Build history of the part. All positions in model axes, mm. Face numbers are marked on the shaded views. A direction names the side the tool comes from. Round coordinates to 2 decimals unless told otherwise and drop trailing zeros. Loops run counter-clockwise (first coordinate to the right, second up) from the corner with the lowest first, then second, coordinate; pieces in that order, holes last.
from build123d import *

# Parameters (mm, degrees)
SKETCH1_W           = 6
SKETCH1_H           = 5
BOSS_EXTRUDE1_DEPTH = 8
SKETCH3_W           = 2
SKETCH3_H           = 5
CUT_EXTRUDE1_DEPTH  = 2
SKETCH4_W           = 2
SKETCH4_H           = 2
CUT_EXTRUDE2_DEPTH  = 1
SKETCH5_W           = 6
SKETCH5_H           = 5
CUT_EXTRUDE3_DEPTH  = 2
SKETCH6_W           = 2
SKETCH6_H           = 2
CUT_EXTRUDE4_DEPTH  = 2
CUT_EXTRUDE5_DEPTH  = 1
SKETCH8_W           = 8.535402973
SKETCH8_H           = 3.487061374
CUT_EXTRUDE6_DEPTH  = 1
SKETCH9_W           = 2
SKETCH9_H           = 1
CUT_EXTRUDE7_DEPTH  = 1


with BuildPart() as part:
    # Sketch1 → Boss-Extrude1 (new body)
    with BuildSketch(Plane.XY):
        Rectangle(SKETCH1_W, SKETCH1_H)
    extrude(amount=BOSS_EXTRUDE1_DEPTH)

    # Sketch3 → Cut-Extrude1 (cut)
    with BuildSketch(Plane.XY.offset(8)):
        with Locations((2, 0)):
            Rectangle(SKETCH3_W, SKETCH3_H)
    extrude(amount=-CUT_EXTRUDE1_DEPTH, mode=Mode.SUBTRACT)

    # Sketch4 → Cut-Extrude2 (cut)
    with BuildSketch(Plane.XY.offset(8)):
        with Locations((0, 1.5)):
            Rectangle(SKETCH4_W, SKETCH4_H)
    extrude(amount=-CUT_EXTRUDE2_DEPTH, mode=Mode.SUBTRACT)

    # Sketch5 → Cut-Extrude3 (cut)
    with BuildSketch(Plane(origin=(0, 2.5, 0), x_dir=(1, 0, 0), z_dir=(0, 1, 0))):
        with Locations((0, -3.5)):
            Rectangle(SKETCH5_W, SKETCH5_H)
    extrude(amount=-CUT_EXTRUDE3_DEPTH, mode=Mode.SUBTRACT)

    # Sketch6 → Cut-Extrude4 (cut)
    with BuildSketch(Plane(origin=(0, 0.5, 0), x_dir=(1, 0, 0), z_dir=(0, 1, 0))):
        with Locations((2, -5)):
            Rectangle(SKETCH6_W, SKETCH6_H)
    extrude(amount=-CUT_EXTRUDE4_DEPTH, mode=Mode.SUBTRACT)

    # Sketch7 → Cut-Extrude5 (cut)
    with BuildSketch(Plane(origin=(0, 0.5, 0), x_dir=(1, 0, 0), z_dir=(0, 1, 0))):
        Polygon((3, -4), (3, -3), (-3, -3), (-3, -6), (1, -6), (1, -4), align=None)
    extrude(amount=-CUT_EXTRUDE5_DEPTH, mode=Mode.SUBTRACT)

    # Sketch8 → Cut-Extrude6 (cut)
    with BuildSketch(Plane(origin=(0, 2.5, 0), x_dir=(1, 0, 0), z_dir=(0, 1, 0))):
        with Locations((-0.885821847, -7.448525998)):
            Rectangle(SKETCH8_W, SKETCH8_H)
    extrude(amount=-CUT_EXTRUDE6_DEPTH, mode=Mode.SUBTRACT)

    # Sketch9 → Cut-Extrude7 (cut)
    with BuildSketch(Plane(origin=(0, 0.5, 0), x_dir=(1, 0, 0), z_dir=(0, 1, 0))):
        with Locations((0, -7.5)):
            Rectangle(SKETCH9_W, SKETCH9_H)
    extrude(amount=-CUT_EXTRUDE7_DEPTH, mode=Mode.SUBTRACT)


solid = part.part
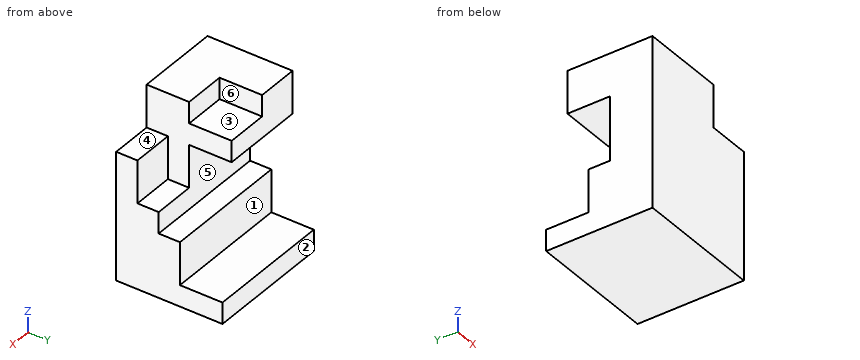
(1) Probe line 1 (Z direction, x = -2.15, y = -0.1); line 2 (Z direction, x = -1.6, y = 1.45); line 3 (X direction, y = -0.95, z = 7.75). List the from-to ranges inside material, lowest first.
Responses:
line 1: z = 0 to 3, 6 to 8
line 2: z = 0 to 1, 6 to 8
line 3: x = -3 to 1
(2) Pin check, flat tips, straight feed: P1, Ø1.6, axis at x = -1, z = 7, coming from the +Y side; P2, Ø1.6, axis at x = 2.5, z = 5, coming from the +Y side; P3, Ø0.5, axis at y = 1, z = 7.5, coming from the +X side. Stop position of each tip, or through.
Responses:
P1: stops at y = 1.5
P2: stops at y = -1.5
P3: stops at x = -1
(3) Which spindle directions (+Z, -Z, +X, -X, +Y, -Y) get a long thin tool onto all of the face, cutting with end or side? Do the marked faces 1, 2 and 3. Say none if no direction does.
Responses:
face 1: +X, -X, +Y
face 2: +Z, -Z, +X, -X, +Y
face 3: +Z, +X, +Y
(4) Slice it at B-B on x = 2.35. List the corners of the cut face in (y, z), plus the area to 3 significant figures.
Responses:
outline: (-2.5, 0) - (2.5, 0) - (2.5, 1) - (0.5, 1) - (0.5, 3) - (-0.5, 3) - (-0.5, 4) - (-1.5, 4) - (-1.5, 6) - (-2.5, 6) - close
area: 15.0 mm2
(5) Slice it at A-A on y = 0.9. List the corners of the cut face in (x, z).
Responses:
outline: (-3, 0) - (3, 0) - (3, 1) - (-3, 1) - close; (-3, 6) - (1, 6) - (1, 7) - (-1, 7) - (-1, 8) - (-3, 8) - close
(6) Slice it at D-D on z = 3.25. List the corners of the cut face in (x, y).
Responses:
outline: (-3, -2.5) - (3, -2.5) - (3, -0.5) - (-3, -0.5) - close
(7) Slice it at C-C on y = 0.3. List the corners of the cut face in (x, z), plus the area to 3 significant figures.
Responses:
outline: (-3, 0) - (3, 0) - (3, 3) - (-3, 3) - close; (-3, 6) - (1, 6) - (1, 7) - (-1, 7) - (-1, 8) - (-3, 8) - close
area: 24.0 mm2
(8) Pull direction Z, two halves, no side cores. Call the marked faces 4, 5 and 6: +Z half, -Z half, draft (parallel to the pull), parting line (faces both ways), or undercut.
Responses:
face 4: +Z half
face 5: undercut
face 6: draft
